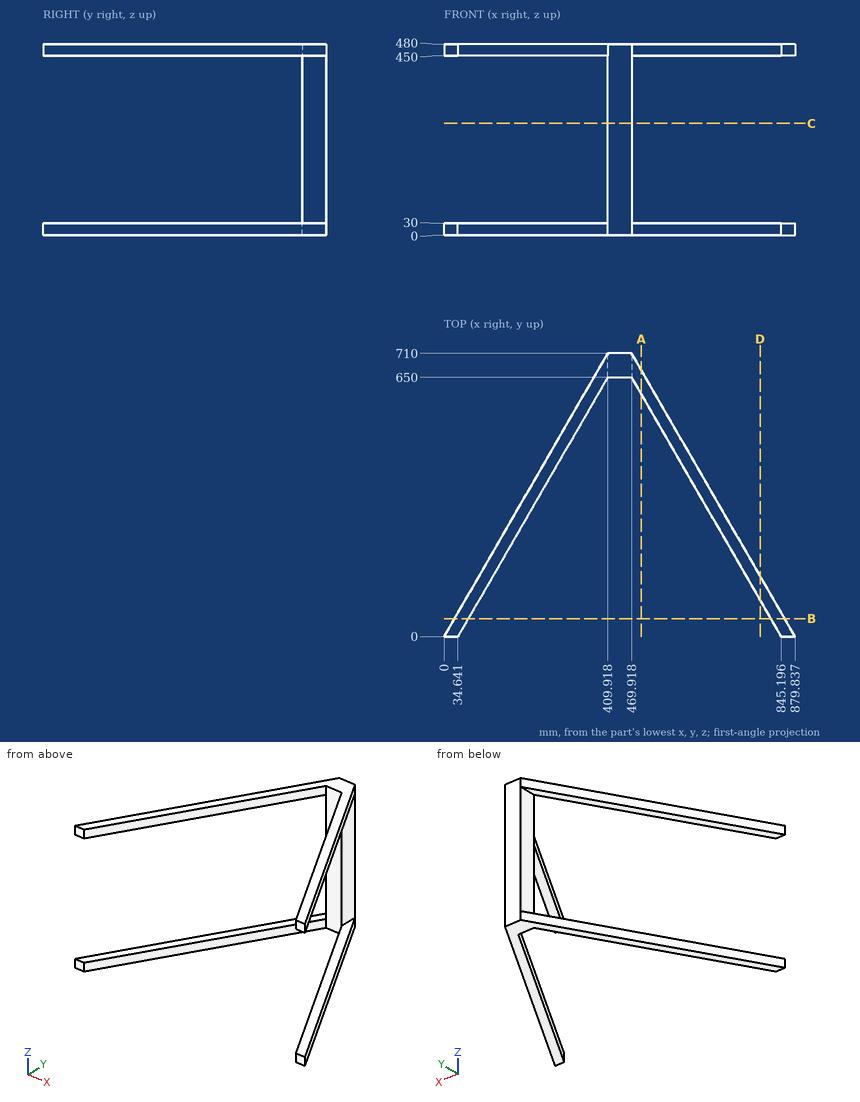
Input: dimensioned drawing with shaded views. Units: mm. Origin: part minimum x, y, z. Round coordinates to 2 decimals unless told otherwise and drop trailing zeros. Loops run counter-clockwise (first coordinate to the right, second up) from the corner with the lowest first, then second, coordinate; pieces in that order, holes last. Notation, with made-up numbers: (8.25, -14) -> (51.25, -14) arc R27 cw to (51.25, 4) -> close; hole circle Ø11 at (-35, 13). An arc over 180 degrees is marked (long way). One line per item, written item: value.
(1) Pin query (flat end, axial travel): pin 1 (18 mm diameter, centred on y = 681.5, z = 187.5, fed in from -X). Return the tip coordinate at first contact, or that it passes through.
Geometry check:
pin 1: x = 409.92
(2) Section C-C (z = 281). Return the cut outline in (x, y).
Geometry check:
outline: (409.92, 650) -> (469.92, 650) -> (469.92, 710) -> (409.92, 710) -> close
(3) Section B-B (y = 45). Return the cut outline in (x, z) (1 decimal), plus the area to 3 significant figures.
Geometry check:
outline: (26, 0) -> (60.6, 0) -> (60.6, 30) -> (26, 30) -> close; (26, 450) -> (60.6, 450) -> (60.6, 480) -> (26, 480) -> close; (819.2, 0) -> (853.9, 0) -> (853.9, 30) -> (819.2, 30) -> close; (819.2, 450) -> (853.9, 450) -> (853.9, 480) -> (819.2, 480) -> close
area: 4,160 mm2
(4) Section D-D (x = 792.5). Return the cut outline in (y, z), plus the area to 3 significant figures.
Geometry check:
outline: (91.27, 0) -> (151.27, 0) -> (151.27, 30) -> (91.27, 30) -> close; (91.27, 450) -> (151.27, 450) -> (151.27, 480) -> (91.27, 480) -> close
area: 3,600 mm2
(5) Section A-A (x = 494.5). Return the cut outline in (y, z), plus the area to 3 significant figures.
Geometry check:
outline: (607.42, 0) -> (667.42, 0) -> (667.42, 30) -> (607.42, 30) -> close; (607.42, 450) -> (667.42, 450) -> (667.42, 480) -> (607.42, 480) -> close
area: 3,600 mm2
(6) Material intervals for line 1 (Z direction, x = 497.5, y = 618); line 2 (Y direction, x = 672.5, z = 452.5), sorted ascending. Write a range as [from, to].
Geometry check:
line 1: [0, 30], [450, 480]
line 2: [299.12, 359.12]
